Read the model definition and answer for the solid it produces. Units are mm, in the model's axes. A direction names the side the tool comes from. Give positions to 0.01 mm unless a question says otherwise; leave off trailing zeros. Order: outer loops, then holes, each group sorted by start corner. A loop starts at its lowest first (then second) coordinate and runs counter-clockwise, first axis right, second up.
```python
from build123d import *

# Parameters (mm, degrees)
BOSS_EXTRUDE1_DEPTH = 6
CUT_EXTRUDE1_DEPTH  = 5


with BuildPart() as part:
    # Sketch1 → Boss-Extrude1 (new body)
    with BuildSketch(Plane(origin=(0, 0, 0), x_dir=(1, 0, 0), z_dir=(0, 1, 0))):
        with BuildLine():
            ThreePointArc((-3.614057951, 9.714230186), (0, 12), (3.614057951, 9.714230186))
            ThreePointArc((3.614057951, 9.714230186), (5.450234482, 7.501604203), (8.121976593, 6.439035579))
            ThreePointArc((8.121976593, 6.439035579), (11.412678196, 3.708203932), (10.355587244, -0.43531115))
            ThreePointArc((10.355587244, -0.43531115), (8.818664639, -2.865357836), (8.633715541, -5.734687343))
            ThreePointArc((8.633715541, -5.734687343), (7.053423028, -9.708203932), (2.78604694, -9.983267272))
            ThreePointArc((2.78604694, -9.983267272), (0, -9.272492736), (-2.78604694, -9.983267272))
            ThreePointArc((-2.78604694, -9.983267272), (-7.053423028, -9.708203932), (-8.633715541, -5.734687343))
            ThreePointArc((-8.633715541, -5.734687343), (-8.818664639, -2.865357836), (-10.355587244, -0.43531115))
            ThreePointArc((-10.355587244, -0.43531115), (-11.412678196, 3.708203932), (-8.121976593, 6.439035579))
            ThreePointArc((-8.121976593, 6.439035579), (-5.450234482, 7.501604203), (-3.614057951, 9.714230186))
        make_face()
    extrude(amount=BOSS_EXTRUDE1_DEPTH)

    # Sketch2 → Cut-Extrude1 (cut)
    with BuildSketch(Plane(origin=(0, 6, 0), x_dir=(1, 0, 0), z_dir=(0, 1, 0))):
        Polygon((-5.1, 2.944486373), (-5.1, -2.944486373), (0, -5.888972746), (5.1, -2.944486373), (5.1, 2.944486373), (0, 5.888972746), align=None)
    extrude(amount=-CUT_EXTRUDE1_DEPTH, mode=Mode.SUBTRACT)


solid = part.part
```
1) Consider L1, parallel to Y at x = 1.25, z = -4; L2, parallel to X at y = 1.75, z = -3; L3, parallel to X at y = 1.65, z = 4.75. Determine where each line is inside the solid, lowest interval first.
Final values:
L1: y = 0 to 1
L2: x = -11.57 to -5, 5 to 11.57
L3: x = -8.53 to -1.97, 1.97 to 8.53
2) The part is cut by section A-A on y = 2.75. Determine the outline of the cut face in (x, z), and give its area (3 significant figures).
Final values:
outline: (-10.36, 0.44) arc R4 ccw to (-8.12, -6.44) arc R5.82 cw to (-3.61, -9.71) arc R4 ccw to (3.61, -9.71) arc R5.82 cw to (8.12, -6.44) arc R4 ccw to (10.36, 0.44) arc R5.82 cw to (8.63, 5.73) arc R4 ccw to (2.79, 9.98) arc R5.82 cw to (-2.79, 9.98) arc R4 ccw to (-8.63, 5.73) arc R5.82 cw to start; hole (-5.1, -2.94) - (0, -5.89) - (5.1, -2.94) - (5.1, 2.94) - (0, 5.89) - (-5.1, 2.94) - close
area: 270 mm2
3) The part is cut by section C-C on y = 0.65. Determine the outline of the cut face in (x, z).
Final values:
outline: (-10.36, 0.44) arc R4 ccw to (-8.12, -6.44) arc R5.82 cw to (-3.61, -9.71) arc R4 ccw to (3.61, -9.71) arc R5.82 cw to (8.12, -6.44) arc R4 ccw to (10.36, 0.44) arc R5.82 cw to (8.63, 5.73) arc R4 ccw to (2.79, 9.98) arc R5.82 cw to (-2.79, 9.98) arc R4 ccw to (-8.63, 5.73) arc R5.82 cw to start
4) The part is cut by section D-D on x = -1.25. Determine the outline of the cut face in (y, z), and give its area (3 significant figures).
Final values:
outline: (0, -11.8) - (6, -11.8) - (6, -5.17) - (1, -5.17) - (1, 5.17) - (6, 5.17) - (6, 9.41) - (0, 9.41) - close
area: 75.6 mm2
5) The part is cut by section B-B on z = -0.75. Determine the outline of the cut face in (x, y), and give its area (3 significant figures).
Final values:
outline: (-11.22, 0) - (11.22, 0) - (11.22, 6) - (5.1, 6) - (5.1, 1) - (-5.1, 1) - (-5.1, 6) - (-11.22, 6) - close
area: 83.6 mm2
6) Given pin 1 (8 mm diameter, centred on x = 0, z = -1, fed in from +Y), flat-ended and moving along its own axis, determine where the tip first touches the part or whether it passes through.
Final values:
pin 1: stops at y = 1
7) A tool of negligible diameter and unlimited length cuts with its end or side. For faces 5 (the face through (-11.43, 2.96, -3.65)), 6 (the face through (2.586, 3.535, -4.396)), from which of +Z, -Z, +X, -X, +Y, -Y can it reach the whole face along a straight path? Write none if from no direction.
Final values:
face 5: -X, +Y, -Y
face 6: +Y
8) For a pull along Z with two mould halves and no side action, classify faces 1 (the face through (-5.48, 2.96, -7.48)), 2 (the face through (5.1, 4, 0)), 3 (the face through (0, 1, 0)), 4 (the face through (11.39, 2.96, -3.77)) as released by +Z, released by -Z, zero draft, split by the parting line, or undercut.
Final values:
face 1: released by -Z
face 2: undercut
face 3: undercut
face 4: split by the parting line
